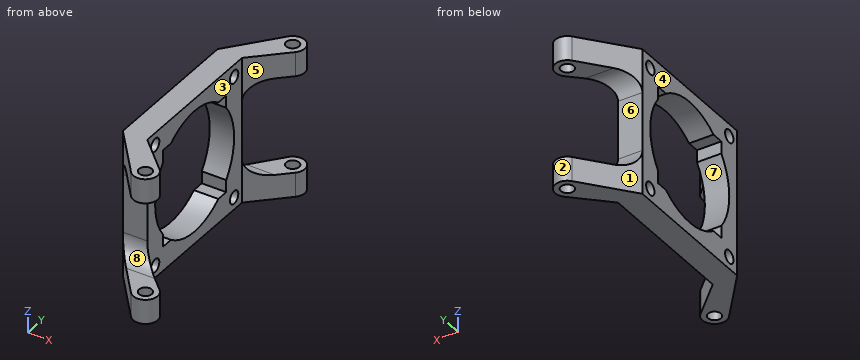
```python
from build123d import *

# Parameters (mm, degrees)
SKETCH_1_W          = 10
SKETCH_1_H          = 40
SKETCH_1_H_2        = 10
SKETCH_1_R          = 5
SKETCH_1_R_2        = 2.65
EXTRUDE_1_DEPTH     = 10
SKETCH_1_5_W        = 10
SKETCH_1_5_H        = 10
EXTRUDE_2_DEPTH     = 50
EXTRUDE_START       = 50
SKETCH_1_6_R        = 5
SKETCH_1_6_R_2      = 2.65
SKETCH_1_6_W        = 10
SKETCH_1_6_H        = 10
SKETCH_1_6_H_2      = 40
EXTRUDE_3_DEPTH     = 10
SKETCH_2_R          = 25
CUT_EXTRUDE_1_DEPTH = 118.763491796
SKETCH_3_R          = 2.65
CUT_EXTRUDE_2_DEPTH = 117.052746628
FILLET_1_R          = 8


with BuildPart() as part:
    # 草图1 → 凸台-拉伸1 (new body)
    with BuildSketch(Plane.XY):
        with Locations((-15, -46.6)):
            Rectangle(SKETCH_1_W, SKETCH_1_H)
        with Locations((-15, -21.6)):
            Rectangle(SKETCH_1_W, SKETCH_1_H_2)
        with BuildLine():
            Line((-3.873829785, 3.161240705), (-20, -16.6))
            Line((-20, -16.6), (-10, -16.6))
            Line((-10, -16.6), (3.472226939, -3.597727072))
            ThreePointArc((3.472226939, -3.597727072), (-3.38544422, -3.679506412), (-3.873829785, 3.161240705))
        make_face()
        Circle(SKETCH_1_R)
        Circle(SKETCH_1_R_2, mode=Mode.SUBTRACT)
        with Locations((-15, -71.6)):
            Rectangle(SKETCH_1_W, SKETCH_1_H_2)
        with BuildLine():
            Line((-10, -76.6), (-20, -76.6))
            Line((-20, -76.6), (-3.873829785, -96.361240705))
            ThreePointArc((-3.873829785, -96.361240705), (-3.587719738, -89.717433837), (3.044640112, -89.233872595))
            Line((3.044640112, -89.233872595), (-10, -76.6))
        make_face()
        with Locations((0, -93.2)):
            Circle(SKETCH_1_R)
        with Locations((0, -93.2)):
            Circle(SKETCH_1_R_2, mode=Mode.SUBTRACT)
    extrude(amount=EXTRUDE_1_DEPTH)

    # 草图1<5> → 凸台-拉伸2 (add)
    with BuildSketch(Plane.XY):
        with Locations((-15, -21.6)):
            Rectangle(SKETCH_1_5_W, SKETCH_1_5_H)
        with Locations((-15, -71.6)):
            Rectangle(SKETCH_1_5_W, SKETCH_1_5_H)
    extrude(amount=EXTRUDE_2_DEPTH)

    # 草图1<6> → 凸台-拉伸3 (add)
    with BuildSketch(Plane.XY.offset(EXTRUDE_START)):
        Circle(SKETCH_1_6_R)
        Circle(SKETCH_1_6_R_2, mode=Mode.SUBTRACT)
        with BuildLine():
            Line((-3.873829785, 3.161240705), (-20, -16.6))
            Line((-20, -16.6), (-10, -16.6))
            Line((-10, -16.6), (3.472226939, -3.597727072))
            ThreePointArc((3.472226939, -3.597727072), (-3.38544422, -3.679506412), (-3.873829785, 3.161240705))
        make_face()
        with Locations((-15, -21.6)):
            Rectangle(SKETCH_1_6_W, SKETCH_1_6_H)
        with Locations((-15, -46.6)):
            Rectangle(SKETCH_1_6_W, SKETCH_1_6_H_2)
        with Locations((-15, -71.6)):
            Rectangle(SKETCH_1_6_W, SKETCH_1_6_H)
        with Locations((0, -93.2)):
            Circle(SKETCH_1_6_R)
        with Locations((0, -93.2)):
            Circle(SKETCH_1_6_R_2, mode=Mode.SUBTRACT)
        with BuildLine():
            Line((-10, -76.6), (-20, -76.6))
            Line((-20, -76.6), (-3.873829785, -96.361240705))
            ThreePointArc((-3.873829785, -96.361240705), (-3.587719738, -89.717433837), (3.044640112, -89.233872595))
            Line((3.044640112, -89.233872595), (-10, -76.6))
        make_face()
    extrude(amount=EXTRUDE_3_DEPTH)

    # 草图2 → 切除-拉伸1 (cut, through all)
    with BuildSketch(Plane.ZY.offset(20)):
        with Locations((30, -46.6)):
            Circle(SKETCH_2_R)
    extrude(amount=-CUT_EXTRUDE_1_DEPTH, mode=Mode.SUBTRACT)

    # 草图3 → 切除-拉伸2 (cut, through all)
    with BuildSketch(Plane(origin=(-10, 0, 0), x_dir=(0, 0, -1), z_dir=(1, 0, 0))):
        with Locations(Location((-55, -21.6, 0), (0, 0, 90))):
            Circle(SKETCH_3_R)
        with Locations(Location((-5, -21.6, 0), (0, 0, 90))):
            Circle(SKETCH_3_R)
        with Locations(Location((-55, -71.6, 0), (0, 0, 90))):
            Circle(SKETCH_3_R)
        with Locations(Location((-5, -71.6, 0), (0, 0, 90))):
            Circle(SKETCH_3_R)
    extrude(amount=-CUT_EXTRUDE_2_DEPTH, mode=Mode.SUBTRACT)

    # 圆角1
    fillet_1_edges = [part.edges().sort_by_distance(p)[0] for p in [
        (-15, -16.6, 10),
        (-15, -16.6, 50),
        (-15, -76.6, 10),
        (-15, -76.6, 50),
    ]]
    fillet(fillet_1_edges, radius=FILLET_1_R)


solid = part.part
```
Check sheet for the modelled part. Datum: model origin and axes. Units: mm. Face numbers are marked on the shaded views. A direction names the side the tool comes from. Round coordinates to 2 decimals unless told otherwise and drop trailing zeros. Loops run counter-clockwise (first coordinate to the right, second up) from the corner with the lowest first, then second, coordinate; pieces in that order, holes last. Notation, with made-up numbers: M 80.5,61.25 L 128.5,61.25 A34 ccw 128.5,91.25 Z; hole C 15.25,19 d8. An arc over 180 degrees is marked long. Answer as a JSON object with one key per item and string values.
1. Gauge pin test, flat ends, axial feed: P1, Ø6, axis at y = -21.6, z = 55, coming from the +X side; P2, Ø10, axis at y = -72, z = 54, coming from the +X side; P3, Ø4, axis at x = -17, z = 40, coming from the +Y side. Record the tip position at first contact, or that the pin passes through.
Reply:
{"P1": "stops at x = -10", "P2": "stops at x = -9.59", "P3": "stops at y = -16.6"}
2. Section check B-B (y = -54.5). Record the boundary of the cut face in (x, z).
Reply:
{"outline": "M -20,0 L -10,0 L -10,6.28 L -20,6.28 Z; M -20,53.72 L -10,53.72 L -10,60 L -20,60 Z"}
3. Scan lines: line 1 (Y direction, x = -1.75, z = 53); line 2 (Z direction, x = -11, y = -69.5); line 3 (Z direction, x = -13, y = -84.5). Record each from-to range of solid material in increasing order.
Reply:
{"line 1": "y = -97.88 to -95.19, -91.21 to -84.59, -8.64 to -1.99, 1.99 to 4.68", "line 2": "z = 0 to 3.38, 6.62 to 19.97, 40.03 to 53.38, 56.62 to 60", "line 3": "z = 0 to 10, 50 to 60"}
4. Section check C-C (x = -5.5). Record the boundary of the cut face in (y, z), plus the area to 3 significant figures.
Reply:
{"outline": "M -94.37,0 L -80.96,0 L -80.96,10.88 A8 cw -84.6,10 L -94.37,10 Z; M -94.37,50 L -84.6,50 A8 cw -80.96,49.12 L -80.96,60 L -94.37,60 Z; M -12.26,0 L 1.17,0 L 1.17,10 L -8.6,10 A8 cw -12.26,10.88 Z; M -12.26,49.12 A8 cw -8.6,50 L 1.17,50 L 1.17,60 L -12.26,60 Z", "area": "541 mm²"}
5. Mould release check, pull along Y, two halves, no side actions. Record for the marked faces 1, 2, 3 and 4: pulls with the +Y half, pulls with the -Y half, needs draft (parallel to the pull), parting line crosses it, or undercut.
Reply:
{"face 1": "pulls with the +Y half", "face 2": "undercut", "face 3": "undercut", "face 4": "needs draft"}
6. Section check A-A (z = 30). Record the boundary of the cut face in (x, y), plus the area to 3 significant figures.
Reply:
{"outline": "M -20,-76.6 L -10,-76.6 L -10,-71.6 L -20,-71.6 Z; M -20,-21.6 L -10,-21.6 L -10,-16.6 L -20,-16.6 Z", "area": "100 mm²"}
7. Section check D-D (y = 0). Record the boundary of the cut face in (x, z).
Reply:
{"outline": "M -6.45,0 L -2.65,0 L -2.65,10 L -6.45,10 Z; M -6.45,50 L -2.65,50 L -2.65,60 L -6.45,60 Z; M 2.65,0 L 5,0 L 5,10 L 2.65,10 Z; M 2.65,50 L 5,50 L 5,60 L 2.65,60 Z"}
8. Access from +Z, -Z, +X, -X, +Y, -Y to the whole of each face (thin tool, end or side, straight path). Record for the marked faces 5, 6, 7 and 8.
Reply:
{"face 5": "+Z, -Z, +X", "face 6": "+X, -X, +Y", "face 7": "+X, -X", "face 8": "+X, -X, -Y"}
